Input: part model. Units: mm. Frame: model coordinates. A direction names the side the tool comes from. Coordinates: 2 decimals unless noted, no trailing zeros. Write each loop counter-clockwise with the first axis right and the second up, starting at its lowest first coordinate (ties: lowest second). Pieces come first, ordered by that corner, then holes. Notation, with made-up numbers: (26.25, 82.5) -> (45.25, 82.5) arc R22 ccw to (45.25, 119.5) -> close; hole circle Ø2 at (62.25, 84.5). An arc over 180 degrees is marked (long way). Use one line per item in the form item = value. Start each with the question number.
(1) Ray query, line 1 along X through (y, z) = (-30, 15); line 2 along X through (y, z) = (-21, 28.5); line 3 along Y through (x, z) = (56, 34). Return the intervals inside material, ascending.
(2) Cut plane D-D on y = -10. Return the cut outline in (x, z), plus the area to 3 significant figures.
(3) First-contact query: pin 1 (1 mm diameter, centred on x = 29.5, z = 43, fed in from +Y). Flat tip, straight axial feed; report the tip coordinate or a pass-through.
(4) Cut plane A-A on y = -29.5. Return the cut outline in (x, z), plus the area to 3 significant figures.
(5) Pull-direction query (X, two-part tool) for faces 4 (the face through (44, -54, 0)), 5 (the face through (85.07, -10.386, 38.872)), 6 (the face through (-10, -30, 30)), 7 (the face through (100, -30, 30)); classes: released by +X, released by -X, zero draft, split by the parting line, or undercut.
(6) Cut plane B-B on z = 22. Return the cut outline in (x, y), plus the area to 3 significant figures.
(7) Set-up query: faces 1 (the face through (4.93, -10.386, 21.128)), 2 (the face through (44, -54, 60)), 3 (the face through (80, -15, 30)). Return all of +Z, -Z, +X, -X, +Y, -Y with unobstructed straight access to the full face (end or side cutting, diameter ignored); none if empty.
(8) Cut plane C-C on x = 25.5. Return the cut outline in (y, z).
```python
from build123d import *

# Parameters (mm, degrees)
F1_DEPTH = 60
F4_DEPTH = 10
F3_R     = 10
F5_DEPTH = 10
F6_DEPTH = 25
F7_DEPTH = 1000


with BuildPart() as f1:
    # F0 (on Top) → F1 (new body)
    with BuildSketch(Plane.XY):
        Polygon((0, -50), (0, 0), (-10, 0), (-10, -60), (100, -60), (100, 0), (90, 0), (90, -50), align=None)
    extrude(amount=F1_DEPTH)

    # F2 (on face) → F4 (join)
    with BuildSketch(Plane(origin=(90, 0, 0), x_dir=(0, -1, 0), z_dir=(-1, 0, 0))):
        with BuildLine():
            ThreePointArc((25, 30), (15, 40), (5, 30))
            ThreePointArc((5, 30), (15, 20), (25, 30))
        make_face()
    extrude(amount=F4_DEPTH)

    # F3 (on face) → F5 (join)
    with BuildSketch(Plane.YZ):
        with Locations((-15, 30)):
            Circle(F3_R)
    extrude(amount=F5_DEPTH)

    # F2 (on face) → F6 (cut)
    with BuildSketch(Plane(origin=(90, 0, 0), x_dir=(0, -1, 0), z_dir=(-1, 0, 0))):
        with BuildLine():
            Line((0, 60), (0, 30))
            ThreePointArc((0, 30), (7.0692509723, 49.5256241898), (25, 60))
            Line((25, 60), (0, 60))
        make_face()
        with BuildLine():
            Line((0, 30), (0, 0))
            Line((0, 0), (25, 0))
            ThreePointArc((25, 0), (7.0692509723, 10.4743758102), (0, 30))
        make_face()
    extrude(amount=-F6_DEPTH, mode=Mode.SUBTRACT)

    # F2 (on face) → F7 (cut)
    with BuildSketch(Plane(origin=(90, 0, 0), x_dir=(0, -1, 0), z_dir=(-1, 0, 0))):
        with BuildLine():
            Line((0, 60), (0, 30))
            ThreePointArc((0, 30), (7.0692509723, 49.5256241898), (25, 60))
            Line((25, 60), (0, 60))
        make_face()
        with BuildLine():
            Line((0, 30), (0, 0))
            Line((0, 0), (25, 0))
            ThreePointArc((25, 0), (7.0692509723, 10.4743758102), (0, 30))
        make_face()
    extrude(amount=F7_DEPTH, mode=Mode.SUBTRACT)


solid = f1.part
```
Values:
q1.line_1 = -10 to 0, 90 to 100
q1.line_2 = -10 to 10, 80 to 100
q1.line_3 = -60 to -50
q2.outline = (-10, 7.42) -> (0, 7.42) -> (0, 21.34) -> (10, 21.34) -> (10, 38.66) -> (0, 38.66) -> (0, 52.58) -> (-10, 52.58) -> close; (80, 21.34) -> (90, 21.34) -> (90, 7.42) -> (100, 7.42) -> (100, 52.58) -> (90, 52.58) -> (90, 38.66) -> (80, 38.66) -> close
q2.area = 1,250 mm2
q3.pin_1 = -50
q4.outline = (-10, 0) -> (0, 0) -> (0, 60) -> (-10, 60) -> close; (90, 0) -> (100, 0) -> (100, 60) -> (90, 60) -> close
q4.area = 1,200 mm2
q5.face_4 = zero draft
q5.face_5 = undercut
q5.face_6 = released by -X
q5.face_7 = released by +X
q6.outline = (-10, -60) -> (100, -60) -> (100, -1.07) -> (90, -1.07) -> (90, -9) -> (80, -9) -> (80, -21) -> (90, -21) -> (90, -50) -> (0, -50) -> (0, -21) -> (10, -21) -> (10, -9) -> (0, -9) -> (0, -1.07) -> (-10, -1.07) -> close
q6.area = 2,320 mm2
q7.face_1 = none
q7.face_2 = +Z, +X, -X, +Y, -Y
q7.face_3 = +Z, -Z, +Y
q8.outline = (-60, 0) -> (-50, 0) -> (-50, 60) -> (-60, 60) -> close
